Build history of the part. All positions in model axes, mm. Face numbers are marked on the shaded views. Coordinates: 2 decimals unless noted, no trailing zeros. Loops run counter-clockwise (first coordinate to the right, second up) from the corner with the lowest first, then second, coordinate; pieces in that order, holes last. Notation, with made-up numbers: (0.5, -36.5) - (11.5, -36.5) arc R19 cw to (11.5, -31.5) - close; hole circle Ø11 at (3.25, 27). An arc over 180 degrees is marked (long way). One line per item, written item: value.
```python
from build123d import *

# Parameters (mm, degrees)
SKETCH1_R                = 36
BOSS_EXTRUDE1_DEPTH      = 60
SKETCH2_R                = 30
CUT_EXTRUDE1_DEPTH       = 60
BOSS_EXTRUDE2_START      = -5
BOSS_EXTRUDE2_DEPTH      = 5
BOSS_EXTRUDE4_DEPTH      = 2.5
BOSS_EXTRUDE4_DEPTH_BACK = 2.5
SKETCH7_R                = 2.5
CUT_EXTRUDE2_DEPTH       = 70.300236124


with BuildPart() as part:
    # Sketch1 → Boss-Extrude1 (new body)
    with BuildSketch(Plane.XY):
        Circle(SKETCH1_R)
    extrude(amount=BOSS_EXTRUDE1_DEPTH)

    # Sketch2 → Cut-Extrude1 (cut)
    with BuildSketch(Plane.XY.offset(60)):
        Circle(SKETCH2_R)
    extrude(amount=-CUT_EXTRUDE1_DEPTH, mode=Mode.SUBTRACT)

    # Sketch5 → Boss-Extrude2 (add)
    with BuildSketch(Plane.XY.offset(24).offset(BOSS_EXTRUDE2_START)):
        with BuildLine():
            Line((-32.726136344, 15), (-42.726136344, 15))
            Line((-42.726136344, 15), (-42.726136344, 0))
            Line((-42.726136344, 0), (-42.726136344, -6))
            Line((-42.726136344, -6), (-36.726136344, -6))
            Line((-36.726136344, -6), (-36.726136344, 11.726443556))
            Line((-36.726136344, 11.726443556), (-34.036605611, 11.726443556))
            ThreePointArc((-34.036605611, 11.726443556), (-33.421474703, 13.379276091), (-32.726136344, 15))
        make_face()
    boss_extrude2 = extrude(amount=BOSS_EXTRUDE2_DEPTH)

    # Mirror1: Boss-Extrude2 across plane
    add(boss_extrude2.mirror(Plane.XY.offset(30)))

    # Sketch6 → Boss-Extrude4 (add, two sides: drawn at the far end of the back side and taken through both)
    with BuildSketch(Plane.XY.offset(30).offset(-BOSS_EXTRUDE4_DEPTH_BACK)):
        with BuildLine():
            Line((-36.726136344, 15), (-42.726136344, 15))
            Line((-42.726136344, 15), (-42.726136344, -6))
            Line((-42.726136344, -6), (-32.726136344, -6))
            ThreePointArc((-32.726136344, -6), (-33.421474703, -4.379276091), (-34.036605611, -2.726443556))
            Line((-34.036605611, -2.726443556), (-36.726136344, -2.726443556))
            Line((-36.726136344, -2.726443556), (-36.726136344, 15))
        make_face()
    extrude(amount=BOSS_EXTRUDE4_DEPTH + BOSS_EXTRUDE4_DEPTH_BACK)

    # Sketch7 → Cut-Extrude2 (cut, through all)
    with BuildSketch(Plane.XY.offset(41)):
        with Locations(Location((-39.726136344, -1, 0), (0, 0, 180))):
            Circle(SKETCH7_R)
    extrude(amount=-CUT_EXTRUDE2_DEPTH, mode=Mode.SUBTRACT)


solid = part.part
```
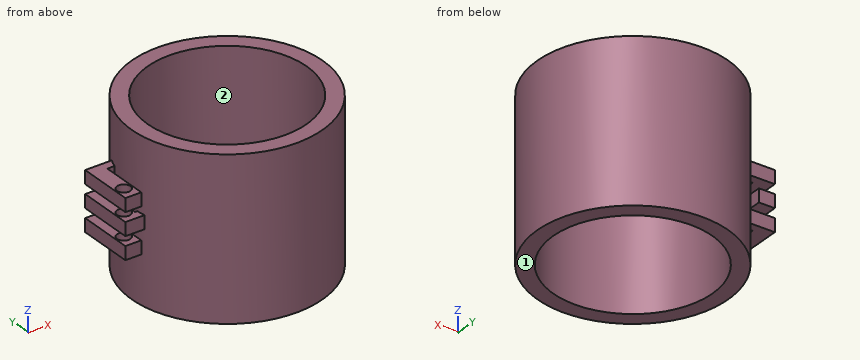
Item 1: Cut at C-C, the plane z = 22. Write the cut outline in (x, y).
Check result:
outline: (-42.73, -6) - (-36.73, -6) - (-36.73, 11.73) - (-34.04, 11.73) arc R36 ccw (long way) to (-32.73, 15) - (-42.73, 15) - close; hole circle Ø5 at (-39.73, -1); hole circle Ø60 at (0, 0)
Item 2: Pull direction Y, two halves, no side cores. Call the marked faces 1 and 2: released by +Y, released by -Y, zero draft, split by the parting line, or undercut.
Check result:
face 1: zero draft
face 2: undercut
Item 3: Cut at B-B, the plane y = -7.5. Write the cut outline in (x, z), then the cut area to 3 significant figures.
Check result:
outline: (-35.21, 0) - (-29.05, 0) - (-29.05, 60) - (-35.21, 60) - close; (29.05, 0) - (35.21, 0) - (35.21, 60) - (29.05, 60) - close
area: 740 mm^2
Item 4: Cut at A-A, the plane x = 0. Write the cut outline in (y, z), then the cut area to 3 significant figures.
Check result:
outline: (-36, 0) - (-30, 0) - (-30, 60) - (-36, 60) - close; (30, 0) - (36, 0) - (36, 60) - (30, 60) - close
area: 720 mm^2
Item 5: Drop flat-ended pins along their axis: P1, Ø2.5, axis at y = 5.5, z = 30.5, coming from the +X side; P2, Ø1, axis at x = -15.5, z = 48.5, coming from the -Y side; P3, Ø1.5, axis at x = -36, z = 21, coming from the +Y side. Give the stop position or say it passes through.
Check result:
P1: stops at x = 35.75
P2: stops at y = -32.73
P3: stops at y = 15
Item 6: Cut at D-D, the plane y = 0. Give the number of separate pieces and of enclosed holes in the cut face, then the cut area to 3 significant figures.
Check result:
separate pieces: 8
enclosed holes: 0
area: 741 mm^2
Item 7: Probe probe 1 along Y at (x, z) = (0, 19); probe 2 along X at (y, z) = (2.5, 50); probe 3 along X at (y, z) = (27, 20.5). List the from-to ranges inside material, lowest first. Write a range as from..to.
Check result:
probe 1: y = -36..-30, 30..36
probe 2: x = -35.91..-29.9, 29.9..35.91
probe 3: x = -23.81..-13.08, 13.08..23.81
